Could you check a few things on this model? Use its own coordinates, in mm. Round coordinates to 2 decimals unless told otherwise and drop trailing zeros. Loops run counter-clockwise (first coordinate to the right, second up) from the corner with the lowest first, then second, coordinate; pieces in that order, holes last. Notation, with made-up numbers: (78.5, 34.25) - (137.5, 34.25) arc R13 cw to (137.5, 42.25) - close; hole circle Ø4 at (3.5, 87.25). An arc over 180 degrees is marked (long way). Answer as CSV lines item,"result". Start each with the question number.
1) Suppose I cut it at A-A, the plane y = -27. Write out the boundary of the cut face in (x, z), then the cut area to 3 significant figures.
2) Please list where these lines run through material, in increasing order: line 1 along Z through (x, y) = (32, -25); line 2 along Y through (x, z) = (0, 11.75).
3) I'm going to push flat-ended pins straight in: pin 1 Ø2 at (y, z) = (-11, 6) entering from -X; pin 2 Ø1.5 at (y, z) = (-13.5, 12) entering from +X; pin 3 Ø1.5 at (y, z) = (13, 11.5) entering from -X; pin 4 Ø8 at (x, z) = (19.5, 6) entering from +Y. Where does each tip first touch, or does it pass through?
4) Suppose I cut it at C-C, the plane z = 9. Write out the boundary of the cut face in (x, y).
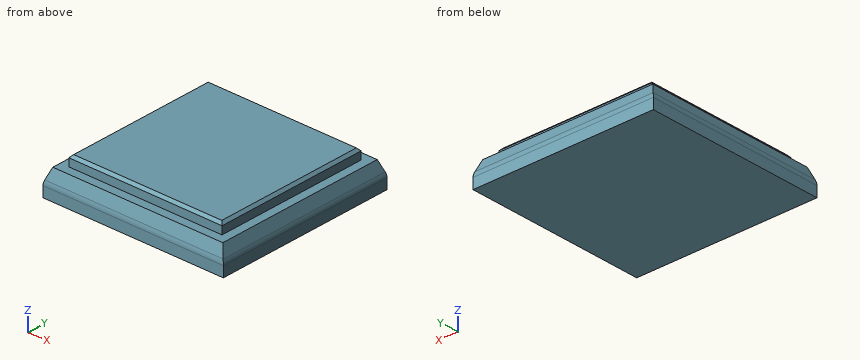
```python
from build123d import *

# Parameters (mm, degrees)
F0_W     = 59.5
F0_H     = 59.5
F1_DEPTH = 14
F0_W_2   = 70
F0_H_2   = 70
F2_DEPTH = 10
F3_SIZE  = 1
F4_SIZE2 = 5
F4_SIZE  = 2
F5_R     = 5


with BuildPart() as f1:
    # F0 (on Top) → F1 (new body)
    with BuildSketch(Plane.XY):
        Rectangle(F0_W, F0_H)
    extrude(amount=F1_DEPTH)

    # F0 (on Top) → F2 (join)
    with BuildSketch(Plane.XY):
        Rectangle(F0_W_2, F0_H_2)
        Rectangle(F0_W, F0_H, mode=Mode.SUBTRACT)
    extrude(amount=F2_DEPTH)

    # F3
    f3_edges = [f1.edges().sort_by_distance(p)[0] for p in [
        (0, -29.75, 14),
        (29.75, 0, 14),
        (0, 29.75, 14),
        (-29.75, 0, 14),
    ]]
    chamfer(f3_edges, length=F3_SIZE)

    # F4
    f4_edges = [f1.edges().sort_by_distance(p)[0] for p in [
        (0, -35, 10),
        (35, 0, 10),
        (0, 35, 10),
        (-35, 0, 10),
    ]]
    f4_side = f1.faces().sort_by_distance((0, -34.010051, 10))[0]
    chamfer(f4_edges, length=F4_SIZE, length2=F4_SIZE2, reference=f4_side)

    # F5
    f5_edges = [f1.edges().sort_by_distance(p)[0] for p in [
        (35, 0, 5),
        (0, -35, 5),
        (-35, 0, 5),
        (0, 35, 5),
    ]]
    fillet(f5_edges, radius=F5_R)


solid = f1.part
```
Filled sheet:
1,outline,"(-35, 0) - (35, 0) - (35, 4.04) arc R5 ccw to (34.64, 5.89) - (33, 10) - (29.75, 10) - (29.75, 13) - (28.75, 14) - (-28.75, 14) - (-29.75, 13) - (-29.75, 10) - (-33, 10) - (-34.64, 5.89) arc R5 ccw to (-35, 4.04) - close"
1,area,"927 mm²"
2,line 1,"0 to 10"
2,line 2,"-29.75 to 29.75"
3,pin 1,"x = -34.91"
3,pin 2,"x = 29.75"
3,pin 3,"x = -29.75"
3,pin 4,"y = 35"
4,outline,"(-33.4, -33.4) - (33.4, -33.4) - (33.4, 33.4) - (-33.4, 33.4) - close"
